```python
from build123d import *

# Parameters (mm, degrees)
SKETCH_R     = 7.5
PAD_DEPTH    = 60
SKETCH001_W  = 5
SKETCH001_H  = 100
POCKET_DEPTH = 4.001
SKETCH002_W  = 10
SKETCH002_H  = 10
PAD001_DEPTH = 1.5
FILLET_R     = 4


with BuildPart() as part:
    # Sketch → Pad (new body, symmetric)
    with BuildSketch(Plane.XZ):
        Circle(SKETCH_R)
    extrude(amount=PAD_DEPTH, both=True)

    # Sketch001 → Pocket (cut, through all)
    with BuildSketch(Plane.XY.offset(-3.5)):
        Rectangle(SKETCH001_W, SKETCH001_H)
    extrude(amount=-POCKET_DEPTH, mode=Mode.SUBTRACT)

    # Sketch002 → Pad001 (join, symmetric)
    with BuildSketch(Plane.XY):
        with Locations((0, -65)):
            Rectangle(SKETCH002_W, SKETCH002_H)
        with Locations((0, 65)):
            Rectangle(SKETCH002_W, SKETCH002_H)
    extrude(amount=PAD001_DEPTH, both=True)

    # Fillet
    fillet_edges = [part.edges().sort_by_distance(p)[0] for p in [
        (-5, 70, 0),
        (5, 70, 0),
        (5, -70, 0),
        (-5, -70, 0),
    ]]
    fillet(fillet_edges, radius=FILLET_R)


solid = part.part
```
Verification items for the finished model (mm, model axes). A direction names the side the tool comes from. Round coordinates to 2 decimals unless told otherwise and drop trailing zeros. Order: outer loops, then holes, each group sorted by start corner. A loop starts at its lowest first (then second) coordinate and runs counter-clockwise, first axis right, second up. Notation, with made-up numbers: (-0.75, 14) -> (47.25, 14) arc R36 cw to (47.25, 48) -> close; hole circle Ø9 at (-21.5, 19). An arc over 180 degrees is marked (long way). Put each result on its own line as item: value. Start each with the question number.
(1) Section check A-A (z = 0). Enter the section's corners in (x, y).
(2) Draft check along X on faces 4 (the face through (0, 50, -5)), 5 (the face through (3.859, -68.797, 0.021)), 6 (the face through (0, -65, 1.5)). Enter one of: +X half, -X half, draft (parallel to the pull), parting line (faces both ways), or undercut.
(3) Tool access check on faces 1 (the face through (-5, 63, 0)), 2 (the face through (0, 65, -1.5)), 3 (the face through (5, 63, 0)). Record the directions out of +Z, -Z, +X, -X, +Y, -Y that give a thin tool (end or side, any length) a straight path to the whole face; none if there is none.
(4) Section check B-B (y = -29.5). Enter the section's corners in (x, z), then the cut area to 3 significant figures.
(5) Material ranges on line 1 along Y through (x, z) = (-0.25, -4); line 2 along Z through (x, y) = (0.25, 12); line 3 along Y through (x, z) = (-5.5, -3), recorded low to high.
(6) Depth check by flat-ended pin: pin 1 Ø2 at (y, z) = (-47, 4.5) entering from +X; pin 2 Ø1.1 at (y, z) = (1.5, -5) entering from +X; pin 3 Ø3.5 at (y, z) = (63, 0.5) entering from +X. Enter the tip coordinate at first touch or a pass-through.
(7) Section check C-C (z = 6). Enter the section's corners in (x, y), then the cut area to 3 significant figures.
Completed:
1. outline: (-7.5, -60) -> (-5, -60) -> (-5, -66) arc R4 ccw to (-1, -70) -> (1, -70) arc R4 ccw to (5, -66) -> (5, -60) -> (7.5, -60) -> (7.5, 60) -> (5, 60) -> (5, 66) arc R4 ccw to (1, 70) -> (-1, 70) arc R4 ccw to (-5, 66) -> (-5, 60) -> (-7.5, 60) -> close
2. face 4: undercut
2. face 5: +X half
2. face 6: draft
3. face 1: +Z, -Z, -X, +Y
3. face 2: -Z, +X, -X, +Y
3. face 3: +Z, -Z, +X, +Y
4. outline: (-2.5, -7.07) -> (-2.5, -3.5) -> (2.5, -3.5) -> (2.5, -7.07) arc R7.5 ccw (long way) to start
4. area: 157 mm2
5. line 1: y = -60 to -50, 50 to 60
5. line 2: z = -3.5 to 7.5
5. line 3: y = -60 to 60
6. pin 1: stops at x = 6.63
6. pin 2: stops at x = 6.04
6. pin 3: stops at x = 5
7. outline: (-4.5, -60) -> (4.5, -60) -> (4.5, 60) -> (-4.5, 60) -> close
7. area: 1,080 mm2
